Input: part model. Units: mm. Frame: model coordinates. Face numbers are marked on the shaded views. Coordinates: 2 decimals unless noted, no trailing zeros.
1) Draft query along Y for the marked faces 1, 2 and 3. Return one class per face: pulls with the +Y half, pulls with the -Y half, needs draft (parallel to the pull), parting line crosses it, or undercut.
2) Pin query (flat end, axial travel): pin 1 Ø1 at (x, z) = (-6.5, 21) entering from +Y; pin 2 Ø7.5 at (x, y) = (0, 0) entering from +Z (3 decimals); pin 3 Ø1 at (y, z) = (-15.5, 36) entering from -X; pin 4 Ø4 at (y, z) = (8, 14.5) entering from +X. Return the tip coordinate at first contact, or that it passes through.
3) Line query: L1, parallel to Y at x = 0, z = 35; L2, parallel to Y at x = 0, z = 31; L3, parallel to X at y = 0, z = 2. Output: solid intervals per line, ascending.
from build123d import *

# Parameters (mm, degrees)
F2_R     = 4.7625
F3_DEPTH = 24.765
F4_R     = 1.5875
F5_DEPTH = 9.525
F7_R     = 7.62


# Not quite as in the source:
# - a fillet or chamfer that OpenCascade refuses, or shapes differently, is made with other operations: its cross-section is extruded or revolved along the edge and cut away or added


with BuildPart() as f1:
    # F0 (on Front) → F1 (revolve)
    with BuildSketch(Plane.XZ):
        Polygon((11.8329105899, 9.1992265151), (26.5666254177, 24.660434838), (31.75, 24.660434838), (31.75, 34.820434838), (12.3952, 34.820434838), (12.3952, 45.72), (0, 45.72), (0, 0), (4.4022302061, 0), (9.0794198883, 6.3097791593), align=None)
        Polygon((11.8329105899, 3.9054930676), (11.8329105899, 9.1992265151), (9.0794198883, 6.3097791593), (4.4022302061, 0), (6.9125830196, 0), align=None)
    revolve(axis=Axis((0, 0, 22.86), (0, 0, -1)))

    # F2 (on face) → F3 (cut)
    with BuildSketch(Plane.XY.offset(45.72)):
        Circle(F2_R)
    extrude(amount=-F3_DEPTH, mode=Mode.SUBTRACT)

    # F4 (on face) → F5 (cut)
    with BuildSketch(Plane(origin=(0, 0, 0), x_dir=(1, 0, 0), z_dir=(0, 0, -1))):
        Circle(F4_R)
    extrude(amount=-F5_DEPTH, mode=Mode.SUBTRACT)

    # F6: fillet of radius 17.3381993495 on 3 edges, made by hand

    # F6_s1 → F6_t2 (revolve)
    with BuildSketch(Plane.XZ):
        with BuildLine():
            ThreePointArc((16.5322882716, 14.130641177), (13.3299473179, 9.4099376621), (11.8329105899, 3.9054930676))
            Line((11.8329105899, 3.9054930676), (11.4878890775, 3.9402122077))
            ThreePointArc((11.4878890775, 3.9402122077), (11.4861466029, 6.5523597914), (11.4861466029, 9.1992265151))
            Line((11.4861466029, 9.1992265151), (11.5818766312, 9.4384486175))
            Line((11.5818766312, 9.4384486175), (16.2812543129, 14.3698632794))
            Line((16.2812543129, 14.3698632794), (16.5322882716, 14.130641177))
        make_face()
    revolve(axis=Axis((0, 0, 9.1992265151), (0, 0, -1)))

    # F6_s3 → F6_t4 (revolve)
    with BuildSketch(Plane.XZ):
        with BuildLine():
            ThreePointArc((21.6021022057, 19.4507827916), (26.2353502113, 22.9140514833), (31.75, 24.660434838))
            Line((31.75, 24.660434838), (31.7019239972, 25.0038499813))
            ThreePointArc((31.7019239972, 25.0038499813), (29.1583127088, 25.007198825), (26.5666254177, 25.007198825))
            Line((26.5666254177, 25.007198825), (26.3155914589, 24.8996569403))
            Line((26.3155914589, 24.8996569403), (21.351068247, 19.6900048939))
            Line((21.351068247, 19.6900048939), (21.6021022057, 19.4507827916))
        make_face()
    revolve(axis=Axis((0, 0, 24.660434838), (0, 0, -1)))

    # F7
    f7_edges = [f1.edges().sort_by_distance(p)[0] for p in [
        (9.372747, 0, 1.952747),
        (-11.832911, 0, 3.905493),
        (-6.912583, 0, 0),
    ]]
    fillet(f7_edges, radius=F7_R)


solid = f1.part
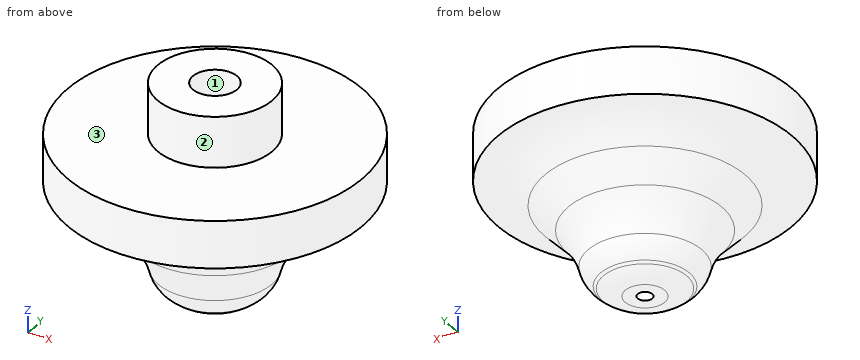
Answer:
1. face 1: undercut
1. face 2: parting line crosses it
1. face 3: needs draft
2. pin 1: stops at y = 23.05
2. pin 2: stops at z = 20.955
2. pin 3: passes through
2. pin 4: stops at x = 17.18
3. L1: y = -12.4 to -4.76, 4.76 to 12.4
3. L2: y = -31.75 to -4.76, 4.76 to 31.75
3. L3: x = -9.43 to -1.59, 1.59 to 9.43
